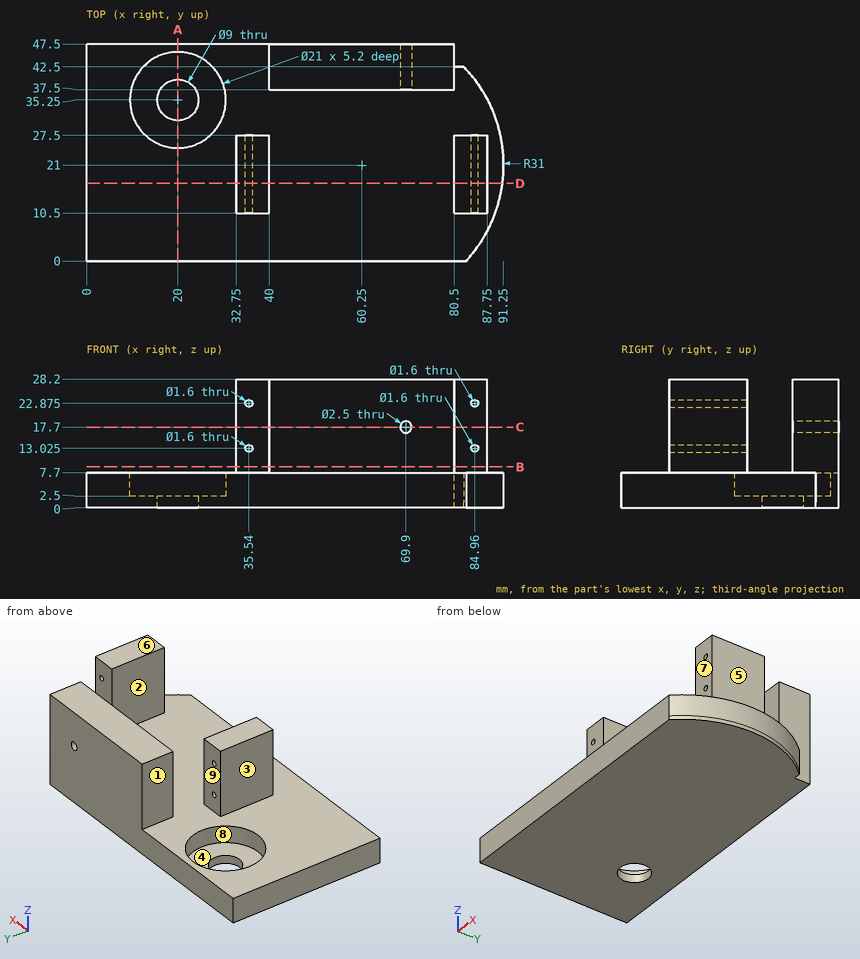
Study the drawing (mm; zero at the part's minimum x, y, z) and answer. A direction names the side the tool comes from. Round coordinates to 2 decimals unless told otherwise and drop trailing zeros. Loops run counter-clockwise (first coordinate to the right, second up) from the corner with the lowest first, then second, coordinate; pieces in that order, holes last. Notation, with made-up numbers: (66, 65) - (94, 65) arc R17 cw to (94, 77) - close; hole circle Ø4 at (40.5, 4.25). An arc over 180 degrees is marked (long way). Use one line per item in the form item = value. Start each with the question number.
1. The part is cut by section C-C on z = 17.7. Determine the outline of the cut face in (x, y), then the cut area to 4 significant figures.
2. The part is cut by section B-B on z = 9. Determine the outline of the cut face in (x, y).
3. A tool of negligible diameter and unlimited length cuts with its end or side. For the marked faces 1, 2, 3, 4 and 5, from which of +Z, -Z, +X, -X, +Y, -Y can it reach the whole face along a straight path? Write none if from no direction.
4. Given pin 1 Ø8 at (y, z) = (41, 15.5) entering from -X; pin 2 Ø8.5 at (y, z) = (18.5, 18) entering from -X; pin 3 Ø5 at (y, z) = (42, 12.5) entering from +X, each flat-ended and moving along its own axis, determine where each tip first touches the part or whether it passes through.
5. Consider line 1 (Z direction, x = 35.54, y = 18.25) (3 decimals); line 2 (Y direction, x = 20, z = 3.7); line 3 (Z direction, x = 69.9, y = 40.5). Determine where each line is inside the solid, lowest interval first. Write a range as [from, to].
6. The part is cut by section D-D on y = 17. Determine the outline of the cut face in (x, z) (3 decimals), then the cut area to 3 significant figures.
7. For a pull along Y with two mould halves and no side action, classify the marked faces 6, 7, 8 and 9 as pulls with the +Y half, pulls with the -Y half, needs draft (parallel to the pull), parting line crosses it, or undercut.
8. The part is cut by section A-A on x = 20. Determine the outline of the cut face in (y, z), then the cut area to 3 significant figures.
Geometry check:
q1.outline = (32.75, 10.5) - (40, 10.5) - (40, 27.5) - (32.75, 27.5) - close; (40, 37.5) - (68.65, 37.5) - (68.65, 47.5) - (40, 47.5) - close; (71.15, 37.5) - (80.5, 37.5) - (80.5, 47.5) - (71.15, 47.5) - close; (80.5, 10.5) - (87.75, 10.5) - (87.75, 27.5) - (80.5, 27.5) - close
q1.area = 626.5 mm^2
q2.outline = (32.75, 10.5) - (40, 10.5) - (40, 27.5) - (32.75, 27.5) - close; (40, 37.5) - (80.5, 37.5) - (80.5, 47.5) - (40, 47.5) - close; (80.5, 10.5) - (87.75, 10.5) - (87.75, 27.5) - (80.5, 27.5) - close
q3.face_1 = +Z, -X, +Y
q3.face_2 = +Z, -Y
q3.face_3 = +Z, -X, +Y, -Y
q3.face_4 = +Z
q3.face_5 = +Z, +X, +Y, -Y
q4.pin_1 = 40
q4.pin_2 = 32.75
q4.pin_3 = 80.5
q5.line_1 = [0, 12.225], [13.825, 22.075], [23.675, 28.2]
q5.line_2 = [0, 24.75], [45.75, 47.5]
q5.line_3 = [0, 16.45], [18.95, 28.2]
q6.outline = (0, 0) - (90.991, 0) - (90.991, 7.7) - (87.75, 7.7) - (87.75, 28.2) - (80.5, 28.2) - (80.5, 7.7) - (40, 7.7) - (40, 28.2) - (32.75, 28.2) - (32.75, 7.7) - (0, 7.7) - close; hole circle Ø1.6 at (35.54, 13.025); hole circle Ø1.6 at (35.54, 22.875); hole circle Ø1.6 at (84.96, 13.025); hole circle Ø1.6 at (84.96, 22.875)
q6.area = 990 mm^2
q7.face_6 = needs draft
q7.face_7 = pulls with the -Y half
q7.face_8 = undercut
q7.face_9 = pulls with the +Y half
q8.outline = (0, 0) - (30.75, 0) - (30.75, 2.5) - (24.75, 2.5) - (24.75, 7.7) - (0, 7.7) - close; (39.75, 0) - (47.5, 0) - (47.5, 7.7) - (45.75, 7.7) - (45.75, 2.5) - (39.75, 2.5) - close
q8.area = 234 mm^2
